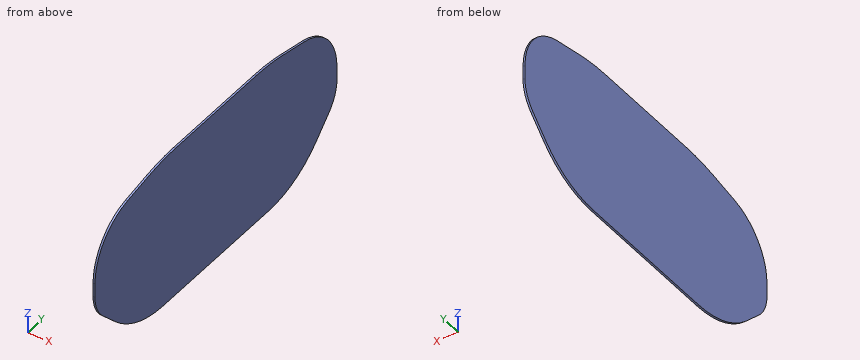
from build123d import *

# Parameters (mm, degrees)
BOSS_EXTRUDE1_DEPTH = 1
FILLET1_R           = 100
FILLET2_R           = 30
FILLET3_R           = 20
FILLET4_R           = 50


with BuildPart() as part:
    # Sketch1 → Boss-Extrude1 (new body)
    with BuildSketch(Plane.YZ):
        Polygon((-40, 40), (40, 40), (90, 30), (90, 0), (90, -10), (60, -40), (-60, -40), (-90, -10), (-90, 0), (-90, 30), align=None)
    extrude(amount=BOSS_EXTRUDE1_DEPTH)

    # Fillet1
    fillet1_edges = [part.edges().sort_by_distance(p)[0] for p in [
        (0.5, -40, 40),
        (0.5, 40, 40),
    ]]
    fillet(fillet1_edges, radius=FILLET1_R)

    # Fillet2
    fillet2_edges = [part.edges().sort_by_distance(p)[0] for p in [
        (0.5, 90, 30),
        (0.5, -90, 30),
    ]]
    fillet(fillet2_edges, radius=FILLET2_R)

    # Fillet3
    fillet3_edges = [part.edges().sort_by_distance(p)[0] for p in [
        (0.5, 90, -10),
        (0.5, -90, -10),
    ]]
    fillet(fillet3_edges, radius=FILLET3_R)

    # Fillet4
    fillet4_edges = [part.edges().sort_by_distance(p)[0] for p in [
        (0.5, 60, -40),
        (0.5, -60, -40),
    ]]
    fillet(fillet4_edges, radius=FILLET4_R)


solid = part.part
Geometry: final body of the model. Coordinates: model frame, mm. Give positions to 0.01 mm unless a question says otherwise; leave off trailing zeros. Loops run counter-clockwise (first coordinate to the right, second up) from the corner with the lowest first, then second, coordinate; pieces in that order, holes last. Notation, with made-up numbers: (66.5, 64) -> (74.5, 64) arc R15 cw to (74.5, 90) -> close; hole circle Ø9 at (75.25, 68.5). An arc over 180 degrees is marked (long way). Put each result on its own line as item: value.
1. Ray query, line 1 along Y through (x, z) = (0.15, -2.5); line 2 along Y through (x, z) = (0.25, 20); line 3 along Z through (x, y) = (0.8, 57). Return the intervals inside material, ascending. Write a range as [from, to].
Taken from the geometry:
line 1: y = [-89.98, 89.98]
line 2: y = [-86.21, 86.21]
line 3: z = [-36.76, 36.6]
2. Cut plane B-B (z = -20). Return the cut outline in (x, y), plus the area to 3 significant figures.
Taken from the geometry:
outline: (0, -80) -> (1, -80) -> (1, 80) -> (0, 80) -> close
area: 160 mm2
3. Cut plane C-C (y = -61). Return the cut outline in (x, z).
Taken from the geometry:
outline: (0, -35.04) -> (1, -35.04) -> (1, 35.8) -> (0, 35.8) -> close
4. Cut plane A-A (x = 0.4). Return the cut outline in (y, z).
Taken from the geometry:
outline: (-90, -1.72) arc R20 ccw to (-84.14, -15.86) -> (-74.64, -25.36) arc R50 ccw to (-39.29, -40) -> (39.29, -40) arc R50 ccw to (74.64, -25.36) -> (84.14, -15.86) arc R20 ccw to (90, -1.72) -> (90, 5.41) arc R30 ccw to (65.88, 34.82) -> (49.71, 38.06) arc R100 ccw to (30.1, 40) -> (-30.1, 40) arc R100 ccw to (-49.71, 38.06) -> (-65.88, 34.82) arc R30 ccw to (-90, 5.41) -> close
